```python
from build123d import *

# Parameters (mm, degrees)
SKETCH1_W           = 80
SKETCH1_H           = 140
BOSS_EXTRUDE1_DEPTH = 3
SKETCH2_W           = 80
SKETCH2_H           = 140
SKETCH2_W_2         = 74
SKETCH2_H_2         = 134
BOSS_EXTRUDE2_DEPTH = 60
FILLET1_R           = 2
FILLET2_R           = 2
SKETCH6_W           = 80
SKETCH6_H           = 140
BOSS_EXTRUDE3_DEPTH = 12
CUT_EXTRUDE1_DEPTH  = 3
SKETCH8_R           = 1.15
CUT_EXTRUDE2_DEPTH  = 6
FILLET3_R           = 3
SKETCH9_W           = 5
SKETCH9_H           = 26
BOSS_EXTRUDE4_DEPTH = 15
SKETCH10_W          = 5
SKETCH10_H          = 26
BOSS_EXTRUDE5_DEPTH = 53
FILLET4_R           = 3
FILLET5_R           = 3
SKETCH12_W          = 8
SKETCH12_H          = 10
BOSS_EXTRUDE6_DEPTH = 19.88
FILLET6_R           = 5
FILLET7_R           = 2
SKETCH13_R          = 2.25
CUT_EXTRUDE3_DEPTH  = 177.504957437
SKETCH14_W          = 8.2
SKETCH14_H          = 5
CUT_EXTRUDE4_DEPTH  = 3
BOSS_EXTRUDE7_DEPTH = 1.35
SKETCH16_W          = 5
SKETCH16_H          = 2.7
CUT_EXTRUDE5_DEPTH  = 3


with BuildPart() as part:
    # Sketch1 → Boss-Extrude1 (new body)
    with BuildSketch(Plane(origin=(0, 0, 0), x_dir=(1, 0, 0), z_dir=(0, 1, 0))):
        with Locations((40, 70)):
            Rectangle(SKETCH1_W, SKETCH1_H)
    extrude(amount=BOSS_EXTRUDE1_DEPTH)

    # Sketch2 → Boss-Extrude2 (add)
    with BuildSketch(Plane(origin=(0, 3, 0), x_dir=(1, 0, 0), z_dir=(0, 1, 0))):
        with Locations((40, 70)):
            Rectangle(SKETCH2_W, SKETCH2_H)
        with Locations((40, 70)):
            Rectangle(SKETCH2_W_2, SKETCH2_H_2, mode=Mode.SUBTRACT)
    extrude(amount=BOSS_EXTRUDE2_DEPTH)

    # Fillet1
    fillet1_edges = [part.edges().sort_by_distance(p)[0] for p in [
        (3, 3, -70),
        (40, 3, -3),
        (77, 3, -70),
        (40, 3, -137),
        (3, 33, -3),
        (77, 33, -3),
        (77, 33, -137),
        (3, 33, -137),
    ]]
    fillet(fillet1_edges, radius=FILLET1_R)

    # Fillet2
    fillet2_edges = [part.edges().sort_by_distance(p)[0] for p in [
        (40, 0, -140),
        (80, 0, -70),
        (40, 0, 0),
        (0, 0, -70),
    ]]
    fillet(fillet2_edges, radius=FILLET2_R)

    # Sketch6 → Boss-Extrude3 (add)
    with BuildSketch(Plane(origin=(0, 63, 0), x_dir=(1, 0, 0), z_dir=(0, 1, 0))):
        with Locations((40, 70)):
            Rectangle(SKETCH6_W, SKETCH6_H)
        with BuildLine():
            Line((15, 128), (65, 128))
            ThreePointArc((65, 128), (67.121320344, 127.121320344), (68, 125))
            Line((68, 125), (68, 15))
            ThreePointArc((68, 15), (67.121320344, 12.878679656), (65, 12))
            Line((65, 12), (15, 12))
            ThreePointArc((15, 12), (12.878679656, 12.878679656), (12, 15))
            Line((12, 15), (12, 125))
            ThreePointArc((12, 125), (12.878679656, 127.121320344), (15, 128))
        make_face(mode=Mode.SUBTRACT)
    extrude(amount=BOSS_EXTRUDE3_DEPTH)

    # Sketch7 → Cut-Extrude1 (cut)
    with BuildSketch(Plane(origin=(0, 75, 0), x_dir=(1, 0, 0), z_dir=(0, 1, 0))):
        with BuildLine():
            Line((6, 137), (74, 137))
            ThreePointArc((74, 137), (76.121320344, 136.121320344), (77, 134))
            Line((77, 134), (77, 6))
            ThreePointArc((77, 6), (76.121320344, 3.878679656), (74, 3))
            Line((74, 3), (6, 3))
            ThreePointArc((6, 3), (3.878679656, 3.878679656), (3, 6))
            Line((3, 6), (3, 134))
            ThreePointArc((3, 134), (3.878679656, 136.121320344), (6, 137))
        make_face()
        with BuildLine():
            Line((12, 131), (68, 131))
            ThreePointArc((68, 131), (70.121320344, 130.121320344), (71, 128))
            Line((71, 128), (71, 12))
            ThreePointArc((71, 12), (70.121320344, 9.878679656), (68, 9))
            Line((68, 9), (12, 9))
            ThreePointArc((12, 9), (9.878679656, 9.878679656), (9, 12))
            Line((9, 12), (9, 128))
            ThreePointArc((9, 128), (9.878679656, 130.121320344), (12, 131))
        make_face(mode=Mode.SUBTRACT)
    extrude(amount=-CUT_EXTRUDE1_DEPTH, mode=Mode.SUBTRACT)

    # Sketch8 → Cut-Extrude2 (cut)
    with BuildSketch(Plane(origin=(0, 72, 0), x_dir=(1, 0, 0), z_dir=(0, 1, 0))):
        with Locations(Location((6.5, 6.5, 0), (0, 0, 270))):
            Circle(SKETCH8_R)
        with Locations(Location((73.5, 6.5, 0), (0, 0, 270))):
            Circle(SKETCH8_R)
        with Locations(Location((73.5, 133.5, 0), (0, 0, 270))):
            Circle(SKETCH8_R)
        with Locations(Location((6.5, 133.5, 0), (0, 0, 270))):
            Circle(SKETCH8_R)
    extrude(amount=-CUT_EXTRUDE2_DEPTH, mode=Mode.SUBTRACT)

    # Fillet3
    # the kernel refuses this fillet: 3 mm, written as the material it takes off along each edge
    with BuildSketch(Plane(origin=(77, 0, -3), x_dir=(1, 0, 0), z_dir=(0, 0, -1))) as fillet3_piece_1:
        with BuildLine():
            CenterArc((1, -2), 2, 0, 90)
            Line((3, -2), (3, 0))
            Line((3, 0), (1, 0))
        make_face()
    revolve(axis=Axis((77, 0, -3), (0, -1, 0)), revolution_arc=90, mode=Mode.SUBTRACT)
    with BuildSketch(Plane(origin=(3, 0, -3), x_dir=(0, 0, 1), z_dir=(1, 0, 0))) as fillet3_piece_2:
        with BuildLine():
            CenterArc((1, -2), 2, 0, 90)
            Line((3, -2), (3, 0))
            Line((3, 0), (1, 0))
        make_face()
    revolve(axis=Axis((3, 0, -3), (0, -1, 0)), revolution_arc=90, mode=Mode.SUBTRACT)
    with BuildSketch(Plane(origin=(77, 0, -137), x_dir=(0, 0, -1), z_dir=(-1, 0, 0))) as fillet3_piece_3:
        with BuildLine():
            CenterArc((1, -2), 2, 0, 90)
            Line((3, -2), (3, 0))
            Line((3, 0), (1, 0))
        make_face()
    revolve(axis=Axis((77, 0, -137), (0, -1, 0)), revolution_arc=90, mode=Mode.SUBTRACT)
    with BuildSketch(Plane(origin=(3, 0, -137), x_dir=(-1, 0, 0), z_dir=(0, 0, 1))) as fillet3_piece_4:
        with BuildLine():
            CenterArc((1, -2), 2, 0, 90)
            Line((3, -2), (3, 0))
            Line((3, 0), (1, 0))
        make_face()
    revolve(axis=Axis((3, 0, -137), (0, -1, 0)), revolution_arc=90, mode=Mode.SUBTRACT)
    with BuildSketch(Plane(origin=(0, 0, -140), x_dir=(1, 0, 0), z_dir=(0, 1, 0)), Plane(origin=(80, 82.5, -140), x_dir=(-1, 0, 0), z_dir=(0, -1, 0)), Plane(origin=(80, 82.5, 0), x_dir=(0, 0, -1), z_dir=(0, -1, 0)), Plane(origin=(0, 0, 0), x_dir=(0, 0, -1), z_dir=(0, 1, 0))) as fillet3_piece_5:
        with BuildLine():
            CenterArc((FILLET3_R, -FILLET3_R), FILLET3_R, 90, 90)
            Line((0, -FILLET3_R), (0, 0))
            Line((0, 0), (FILLET3_R, 0))
        make_face()
    extrude(amount=82.5, mode=Mode.SUBTRACT)

    # Sketch9 → Boss-Extrude4 (add)
    with BuildSketch(Plane.ZY):
        with Locations((-84.5, 42)):
            Rectangle(SKETCH9_W, SKETCH9_H)
    extrude(amount=BOSS_EXTRUDE4_DEPTH)

    # Sketch10 → Boss-Extrude5 (add)
    with BuildSketch(Plane(origin=(0, 0, -87), x_dir=(-1, 0, 0), z_dir=(0, 0, -1))):
        with Locations((12.5, 42)):
            Rectangle(SKETCH10_W, SKETCH10_H)
    extrude(amount=BOSS_EXTRUDE5_DEPTH)

    # Fillet4
    fillet4_edges = [part.edges().sort_by_distance(p)[0] for p in [
        (0, 42, -87),
        (0, 29, -84.5),
        (0, 42, -82),
        (0, 55, -84.5),
    ]]
    fillet(fillet4_edges, radius=FILLET4_R)

    # Fillet5
    fillet5_edges = [part.edges().sort_by_distance(p)[0] for p in [
        (-15, 42, -82),
        (-10, 42, -87),
        (-12.5, 55, -140),
        (-12.5, 29, -140),
    ]]
    fillet(fillet5_edges, radius=FILLET5_R)

    # Sketch12 → Boss-Extrude6 (add)
    with BuildSketch(Plane.XY):
        with Locations((7, 65)):
            Rectangle(SKETCH12_W, SKETCH12_H)
        with Locations((7, 14.67)):
            Rectangle(SKETCH12_W, SKETCH12_H)
    extrude(amount=BOSS_EXTRUDE6_DEPTH)

    # Fillet6
    # the kernel refuses this fillet: 5 mm, written as the material it adds along each edge
    with BuildSketch(Plane(origin=(11, 70, 0), x_dir=(1, 0, 0), z_dir=(0, -1, 0)), Plane(origin=(11, 19.67, 0), x_dir=(1, 0, 0), z_dir=(0, -1, 0))) as fillet6_piece_1:
        with BuildLine():
            CenterArc((FILLET6_R, FILLET6_R), FILLET6_R, 180, 90)
            Line((0, FILLET6_R), (0, 0))
            Line((0, 0), (FILLET6_R, 0))
        make_face()
    extrude(amount=10)
    with BuildSketch(Plane(origin=(3, 70, 0), x_dir=(0, 1, 0), z_dir=(1, 0, 0)), Plane(origin=(11, 9.67, 0), x_dir=(0, -1, 0), z_dir=(-1, 0, 0))) as fillet6_piece_2:
        with BuildLine():
            CenterArc((FILLET6_R, FILLET6_R), FILLET6_R, 180, 90)
            Line((0, FILLET6_R), (0, 0))
            Line((0, 0), (FILLET6_R, 0))
        make_face()
    extrude(amount=8)
    with BuildSketch(Plane(origin=(3, 70, 0), x_dir=(0, 1, 0), z_dir=(1, 0, 0))) as fillet6_piece_3a_section:
        with BuildLine():
            CenterArc((FILLET6_R, FILLET6_R), FILLET6_R, 180, 90)
            Line((0, FILLET6_R), (0, 0))
            Line((0, 0), (FILLET6_R, 0))
        make_face()
    fillet6_piece_3a = extrude(amount=20.5, mode=Mode.PRIVATE)
    fillet6_piece_3a = split(fillet6_piece_3a, bisect_by=Plane(origin=(11, 71.131975571, 1.131975571), z_dir=(1, 0, 0)), keep=Keep.TOP, mode=Mode.PRIVATE)
    with BuildSketch(Plane(origin=(11, 82.5, 0), x_dir=(1, 0, 0), z_dir=(0, -1, 0))) as fillet6_piece_3b_section:
        with BuildLine():
            CenterArc((FILLET6_R, FILLET6_R), FILLET6_R, 180, 90)
            Line((0, FILLET6_R), (0, 0))
            Line((0, 0), (FILLET6_R, 0))
        make_face()
    fillet6_piece_3b = extrude(amount=22.5, mode=Mode.PRIVATE)
    fillet6_piece_3b = split(fillet6_piece_3b, bisect_by=Plane(origin=(12.131975571, 75, 1.131975571), z_dir=(0, -1, 0)), keep=Keep.TOP, mode=Mode.PRIVATE)
    fillet6_piece_3b = split(fillet6_piece_3b, bisect_by=Plane(origin=(12.131975571, 70, 1.131975571), z_dir=(0, 1, 0)), keep=Keep.TOP, mode=Mode.PRIVATE)
    fillet6_piece_3 = fillet6_piece_3a & fillet6_piece_3b
    add(fillet6_piece_3)
    with BuildSketch(Plane(origin=(11, 19.67, 0), x_dir=(1, 0, 0), z_dir=(0, -1, 0))) as fillet6_piece_4a_section:
        with BuildLine():
            CenterArc((FILLET6_R, FILLET6_R), FILLET6_R, 180, 90)
            Line((0, FILLET6_R), (0, 0))
            Line((0, 0), (FILLET6_R, 0))
        make_face()
    fillet6_piece_4a = extrude(amount=22.5, mode=Mode.PRIVATE)
    fillet6_piece_4a = split(fillet6_piece_4a, bisect_by=Plane(origin=(12.131975571, 9.67, 1.131975571), z_dir=(0, -1, 0)), keep=Keep.TOP, mode=Mode.PRIVATE)
    with BuildSketch(Plane(origin=(23.5, 9.67, 0), x_dir=(0, -1, 0), z_dir=(-1, 0, 0))) as fillet6_piece_4b_section:
        with BuildLine():
            CenterArc((FILLET6_R, FILLET6_R), FILLET6_R, 180, 90)
            Line((0, FILLET6_R), (0, 0))
            Line((0, 0), (FILLET6_R, 0))
        make_face()
    fillet6_piece_4b = extrude(amount=20.5, mode=Mode.PRIVATE)
    fillet6_piece_4b = split(fillet6_piece_4b, bisect_by=Plane(origin=(11, 8.538024429, 1.131975571), z_dir=(1, 0, 0)), keep=Keep.TOP, mode=Mode.PRIVATE)
    fillet6_piece_4 = fillet6_piece_4a & fillet6_piece_4b
    add(fillet6_piece_4)

    # Fillet7
    fillet7_edges = [part.edges().sort_by_distance(p)[0] for p in [
        (7, 60, 19.88),
        (7, 70, 19.88),
        (7, 9.67, 19.88),
        (7, 19.67, 19.88),
    ]]
    fillet(fillet7_edges, radius=FILLET7_R)

    # Sketch13 → Cut-Extrude3 (cut, through all)
    with BuildSketch(Plane.ZY.offset(-3)):
        with Locations(Location((4.5, 65, 0), (0, 0, 270))):
            Circle(SKETCH13_R)
        with Locations(Location((15.38, 65, 0), (0, 0, 270))):
            Circle(SKETCH13_R)
        with Locations(Location((4.5, 14.67, 0), (0, 0, 270))):
            Circle(SKETCH13_R)
        with Locations(Location((15.38, 14.67, 0), (0, 0, 270))):
            Circle(SKETCH13_R)
    extrude(amount=-CUT_EXTRUDE3_DEPTH, mode=Mode.SUBTRACT)

    # Sketch14 → Cut-Extrude4 (cut)
    with BuildSketch(Plane.XY):
        with Locations((57.9, 57.5)):
            Rectangle(SKETCH14_W, SKETCH14_H)
    extrude(amount=-CUT_EXTRUDE4_DEPTH, mode=Mode.SUBTRACT)

    # Sketch15 → Boss-Extrude7 (add)
    with BuildSketch(Plane.XZ):
        with BuildLine():
            Line((19.25, -42.75), (60.75, -42.75))
            ThreePointArc((60.75, -42.75), (61.810660172, -43.189339828), (62.25, -44.25))
            Line((62.25, -44.25), (62.25, -95.75))
            ThreePointArc((62.25, -95.75), (61.810660172, -96.810660172), (60.75, -97.25))
            Line((60.75, -97.25), (19.25, -97.25))
            ThreePointArc((19.25, -97.25), (18.189339828, -96.810660172), (17.75, -95.75))
            Line((17.75, -95.75), (17.75, -44.25))
            ThreePointArc((17.75, -44.25), (18.189339828, -43.189339828), (19.25, -42.75))
        make_face()
        with BuildLine():
            Line((21.25, -44.75), (58.75, -44.75))
            ThreePointArc((58.75, -44.75), (59.810660172, -45.189339828), (60.25, -46.25))
            Line((60.25, -46.25), (60.25, -93.75))
            ThreePointArc((60.25, -93.75), (59.810660172, -94.810660172), (58.75, -95.25))
            Line((58.75, -95.25), (21.25, -95.25))
            ThreePointArc((21.25, -95.25), (20.189339828, -94.810660172), (19.75, -93.75))
            Line((19.75, -93.75), (19.75, -46.25))
            ThreePointArc((19.75, -46.25), (20.189339828, -45.189339828), (21.25, -44.75))
        make_face(mode=Mode.SUBTRACT)
    extrude(amount=BOSS_EXTRUDE7_DEPTH)

    # Sketch16 → Cut-Extrude5 (cut)
    with BuildSketch(Plane.XZ):
        with Locations((40, -48.03)):
            Rectangle(SKETCH16_W, SKETCH16_H)
    extrude(amount=-CUT_EXTRUDE5_DEPTH, mode=Mode.SUBTRACT)


solid = part.part
```
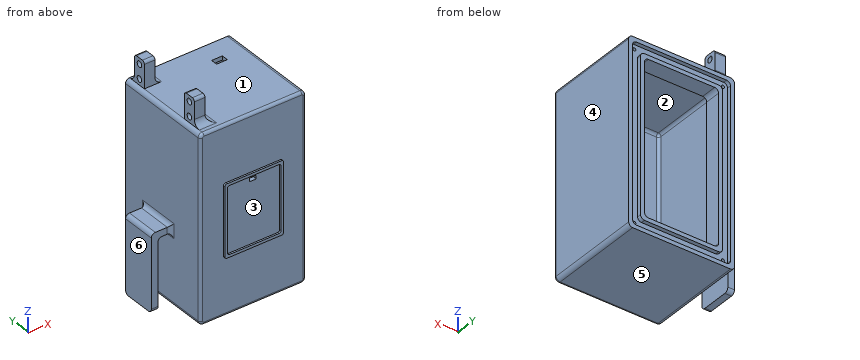
Model file for the job. Use its own axes, mm. Face numbers are marked on the shaded views. A direction names the side the tool comes from. Coordinates: 2 decimals unless noted, no trailing zeros. Write each loop counter-clockwise with the first axis right and the second up, starting at its lowest first coordinate (ties: lowest second). Pieces come first, ordered by that corner, then holes. Notation, with made-up numbers: (29.25, 57.25) - (87.25, 57.25) arc R9 ccw to (87.25, 73.25) - close; hole circle Ø8 at (-4, 34). An arc over 180 degrees is marked (long way). Use a Markdown table: item, result. Add a question column.
Item 1: Drop flat-ended pins along their axis: pin 1 (7 mm diameter, centred on y = 14.67, z = 15.38, fed in from -X); pin 2 (6 mm diameter, centred on y = 70.5, z = -97, fed in from -X); pin 3 (6 mm diameter, centred on x = 22.5, y = 33.5, fed in from +Z). Give the stop position or say it passes through.
Item 2: Two-plate mould, pull along X, no slides. Class the marked faces 3, 4, 5 and 6: pulls with the +X half, pulls with the -X half, needs draft (parallel to the pull), parting line crosses it, or undercut.
Item 3: Band-saw the part on A-A, the plane y = 14.67. Write the cut outline in (x, z), and give its area (3 significant figures).
Item 4: 3-axis set-ups, long thin cutter, end or side, ignore diameter. For the marked faces 1 and 2: which of +Z, -Z, +X, -X, +Y, -Y reach the whole face in a straight line?
Item 5: Band-saw the part on C-C, the plane z = -34. Write the cut outline in (x, y), and give its area (3 significant figures).
Item 6: Drill centre lines: line 1 along X through (y, z) = (40, -127); line 2 along X through (y, z) = (69.2, -133.5); line 3 along Y through (x, z) = (9.5, 4.5). Where is each one in solid material? Low to high.
A:
| question | item | result |
|---|---|---|
| 1 | pin 1 | stops at x = 3 |
| 1 | pin 2 | stops at x = 0 |
| 1 | pin 3 | stops at z = 0 |
| 2 | face 3 | undercut |
| 2 | face 4 | pulls with the +X half |
| 2 | face 5 | needs draft |
| 2 | face 6 | pulls with the -X half |
| 3 | outline | (0, -137) arc R3 ccw to (3, -140) - (77, -140) arc R3 ccw to (80, -137) - (80, -3) arc R3 ccw to (77, 0) - (16, 0) arc R5 cw to (11.82, 2.25) - (3, 2.25) - (3, 0) arc R3 ccw to (0, -3) - close; (3, 6.75) - (11, 6.75) - (11, 13.13) - (3, 13.13) - close; (3, 17.63) - (11, 17.63) - (11, 19.88) - (3, 19.88) - close; hole (3, -135) arc R2 ccw to (5, -137) - (75, -137) arc R2 ccw to (77, -135) - (77, -5) arc R2 ccw to (75, -3) - (5, -3) arc R2 ccw to (3, -5) - close |
| 3 | area | 1,370 mm² |
| 4 | face 1 | +Z, +X |
| 4 | face 2 | none |
| 5 | outline | (0, 2) arc R2 ccw to (2, 0) - (78, 0) arc R2 ccw to (80, 2) - (80, 75) - (77, 75) - (77, 72) - (71, 72) - (71, 75) - (68, 75) - (68, 63) - (77, 63) - (77, 5) arc R2 cw to (75, 3) - (5, 3) arc R2 cw to (3, 5) - (3, 63) - (12, 63) - (12, 75) - (9, 75) - (9, 72) - (3, 72) - (3, 75) - (0, 75) - close |
| 5 | area | 852 mm² |
| 6 | line 1 | x = -15 to -10, 0 to 3, 77 to 80 |
| 6 | line 2 | x = 0 to 5.35, 7.65 to 72.35, 74.65 to 80 |
| 6 | line 3 | y = 9.64 to 12.42, 16.92 to 19.67, 60 to 62.75, 67.25 to 70.03 |
